The model under review builds one solid part; all positions refer to its coordinate system, in mm. A direction names the side the tool comes from. Round coordinates to 2 decimals unless told otherwise and drop trailing zeros. Loops run counter-clockwise (first coordinate to the right, second up) from the corner with the lowest first, then second, coordinate; pieces in that order, holes last. Notation, with made-up numbers: M 6.5,22 L 56.5,22 A24 ccw 56.5,50 Z; hole C 31,46.5 d8. An arc over 180 degrees is marked long. Return JSON: item names as keys, results as strings. Group by question number.
Q1. Consider section C-C (z = -46.5). State the section outline as (x, y) points, and give its area (3 significant figures).
Q2. For faces 1 (the face through (-3, 0, -37)), 2 (the face through (-3, 0, -12)), 3 (the face through (0, 0, -50)), list the 3-axis set-ups (+Z, -Z, +X, -X, +Y, -Y) from which the entire face can be reached by the end or side of a thin tool; tool diameter is ignored.
Q3. Consider section A-A (x = 0). State the section outline as (y, z) points.
Q4. To check wall thickness, follow line 1 along Z through (x, y) = (-2, -4.5); line 2 along X through (y, z) = (-2.25, -23); line 3 along X through (y, z) = (-2.75, -21). State the ranges of each line that lie inside material, in increasing order.
Q5. Clearance check with flat-ended pins moving along their axes: pin 1 Ø2 at (x, z) = (2, -28.5) entering from +Y; pin 2 Ø4 at (x, z) = (4, -10) entering from +Y; pin 3 Ø5 at (y, z) = (1, -12) entering from +X. State where each tip first meets the part, or that it passes through.
Autodesk Inventor part; units mm, degrees
ref_plane "YZ Plane" through (0, 0, 0) normal (1, 0, 0) x (0, 1, 0)
ref_plane "XZ Plane" through (0, 0, 0) normal (0, 1, 0) x (-1, 0, 0)
ref_plane "XY Plane" through (0, 0, 0) normal (0, 0, 1) x (1, 0, 0)
sketch "Sketch1" plane through (0, 0, 0) normal (0, 0, 1) x (1, 0, 0)
  circle A0 centre (0, 0) radius 3
  dimension "d0" = 6
extrude "Extrusion1" add sketch "Sketch1" against normal blind 50
ref_plane "Work Plane1" through (0, 0, -25) normal (0, 0, 1) x (1, 0, 0)
sketch "Sketch2" plane through (0, 0, -25) normal (0, 0, 1) x (1, 0, 0)
  circle A0 centre (0, 0) radius 3
  circle A1 centre (0, 0) radius 3
  circle A2 centre (0, 0) radius 5
  dimension "d3" = 10
extrude "Extrusion2" add sketch "Sketch2" along normal mid plane 1.1
chamfer "Chamfer1" distance 0.5 angle 45 2 edges at (-3, 0, 0) (-3, 0, -50)
properties part number "23-225Z2" material "Stainless Steel"
Values:
{
 "1": {"outline": "C 0,0 d6", "area": "28.3 mm2"},
 "2": {"face 1": "-Z", "face 2": "+Z", "face 3": "-Z, +X, -X, +Y, -Y"},
 "3": {"outline": "M -5,-25.55 L -3,-25.55 L -3,-49.5 L -2.5,-50 L 2.5,-50 L 3,-49.5 L 3,-25.55 L 5,-25.55 L 5,-24.45 L 3,-24.45 L 3,-0.5 L 2.5,0 L -2.5,0 L -3,-0.5 L -3,-24.45 L -5,-24.45 Z"},
 "4": {"line 1": "z = -25.55 to -24.45", "line 2": "x = -1.98 to 1.98", "line 3": "x = -1.2 to 1.2"},
 "5": {"pin 1": "stops at y = 2.83", "pin 2": "stops at y = 2.24", "pin 3": "stops at x = 3"}
}
